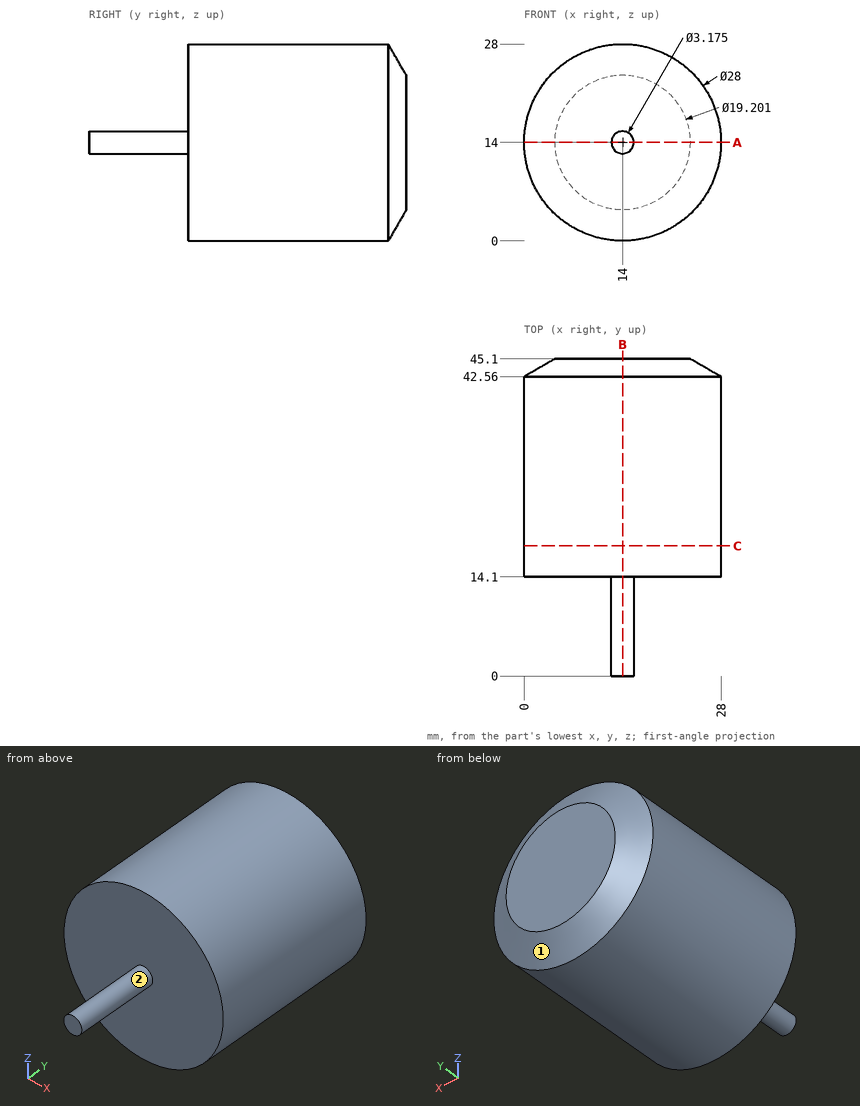
Geometry: see drawing. Coordinates: mm, zero at the bounding-box minimum. A direction names the side the tool comes from. Give positions to 0.01 mm unless a question says otherwise; leave off trailing zeros. Loops run counter-clockwise (first coordinate to the right, second up) from the corner with the lowest first, then second, coordinate; pieces in that order, holes last. Notation, with made-up numbers: (-32, 76) - (18, 76) arc R12 ccw to (18, 98) - close; hole circle Ø1 at (27.5, 22.5). An arc over 180 degrees is marked (long way). Use CSV: the item, a comma, the result in double quotes.
1) Cut plane C-C (y = 18.5). Output: boundary loops of the cut face in (x, z).
Worked out:
outline,"circle Ø28 at (14, 14)"
2) Cut plane B-B (x = 14). Output: boundary loops of the cut face in (y, z), and give its area (3 significant figures).
Worked out:
outline,"(0, 12.41) - (14.1, 12.41) - (14.1, 0) - (42.56, 0) - (45.1, 4.4) - (45.1, 23.6) - (42.56, 28) - (14.1, 28) - (14.1, 15.59) - (0, 15.59) - close"
area,"902 mm^2"
3) Pin query (flat end, axial travel): P1, Ø5, axis at x = 5, z = 24, coming from the -Y side; P2, Ø5, axis at x = 21.5, y = 19.5, coming from the +Z side; P3, Ø8, axis at x = 3, y = 27, coming from the +Z side. Return the tip coordinate at first contact, or that it passes through.
Worked out:
P1,"stops at y = 14.1"
P2,"stops at z = 27.08"
P3,"stops at z = 26.12"
4) Cut plane A-A (z = 14). Output: boundary loops of the cut face in (x, y), and give its area (3 significant figures).
Worked out:
outline,"(0, 14.1) - (12.41, 14.1) - (12.41, 0) - (15.59, 0) - (15.59, 14.1) - (28, 14.1) - (28, 42.56) - (23.6, 45.1) - (4.4, 45.1) - (0, 42.56) - close"
area,"902 mm^2"
5) Line query: line 1 (X direction, y = 40, z = 13.5); line 2 (Y direction, x = 18.5, z = 11.75); line 3 (Z direction, x = 12.75, y = 41). Output: solid intervals per line, ascending.
Worked out:
line 1,"x = 0.01 to 27.99"
line 2,"y = 14.1 to 45.1"
line 3,"z = 0.06 to 27.94"
6) Set-up query: the marked faces 1 and 2. Return all of +Z, -Z, +X, -X, +Y, -Y with unobstructed straight access to the full face (end or side cutting, diameter ignored); none if empty.
Worked out:
face 1,"+Y"
face 2,"-Y"
